Source: CAD feature listing. Evaluate the final solid. Frame: model axes, mm. A direction names the side the tool comes from. Round coordinates to 2 decimals unless told otherwise and drop trailing zeros. Write each loop counter-clockwise with the first axis right and the second up, starting at its lowest first coordinate (ties: lowest second). Pieces come first, ordered by that corner, then holes.
from build123d import *

# Parameters (mm, degrees)
SKETCH1_W           = 30
SKETCH1_H           = 10
BOSS_EXTRUDE1_DEPTH = 6.5
SKETCH3_W           = 13
SKETCH3_H           = 22
CUT_EXTRUDE3_DEPTH  = 20.163767897
SKETCH10_W          = 13
SKETCH10_H          = 10
BOSS_EXTRUDE3_DEPTH = 3
SKETCH12_W          = 22
SKETCH12_H          = 3.25
CUT_EXTRUDE5_DEPTH  = 0.5
SKETCH15_W          = 22
SKETCH15_H          = 3.375
BOSS_EXTRUDE6_DEPTH = 2


with BuildPart() as part:
    # Sketch1 → Boss-Extrude1 (new, symmetric)
    with BuildSketch(Plane.XY):
        Rectangle(SKETCH1_W, SKETCH1_H)
    extrude(amount=BOSS_EXTRUDE1_DEPTH, both=True)

    # Sketch3 → Cut-Extrude3 (cut, through all)
    with BuildSketch(Plane.XZ.offset(5)):
        with Locations((10.5, 0)):
            Rectangle(SKETCH3_W, SKETCH3_H)
    extrude(amount=-CUT_EXTRUDE3_DEPTH, mode=Mode.SUBTRACT)

    # Sketch10 → Boss-Extrude3 (add)
    with BuildSketch(Plane(origin=(4, 0, 0), x_dir=(0, 0, -1), z_dir=(1, 0, 0))):
        Rectangle(SKETCH10_W, SKETCH10_H)
    extrude(amount=BOSS_EXTRUDE3_DEPTH)

    # Sketch12 → Cut-Extrude5 (cut)
    with BuildSketch(Plane(origin=(0, 0, -6.5), x_dir=(-1, 0, 0), z_dir=(0, 0, -1))):
        with Locations((4, 0)):
            Rectangle(SKETCH12_W, SKETCH12_H)
    extrude(amount=-CUT_EXTRUDE5_DEPTH, mode=Mode.SUBTRACT)

    # Sketch15 → Boss-Extrude6 (add)
    with BuildSketch(Plane(origin=(0, 0, -6.5), x_dir=(-1, 0, 0), z_dir=(0, 0, -1))):
        with Locations((4, 3.3125)):
            Rectangle(SKETCH15_W, SKETCH15_H)
    boss_extrude6 = extrude(amount=BOSS_EXTRUDE6_DEPTH)

    # Mirror5: Boss-Extrude6 across plane
    add(boss_extrude6.mirror(Plane.ZX))


solid = part.part
1) Section query C-C on y = 0.25. Return the cut outline in (x, z).
Taken from the geometry:
outline: (-15, -6) - (7, -6) - (7, 6.5) - (-15, 6.5) - close
2) Section query A-A on z = -7. Return the cut outline in (x, y) (3 decimals), then the cut area to 4 significant figures.
Taken from the geometry:
outline: (-15, -5) - (7, -5) - (7, -1.625) - (-15, -1.625) - close; (-15, 1.625) - (7, 1.625) - (7, 5) - (-15, 5) - close
area: 148.5 mm2
3) Material intervals for line 1 (Y direction, x = 3.75, z = -6.5) (3 decimals); line 2 (Z direction, x = 5, y = 1.25), sorted ascending.
Taken from the geometry:
line 1: y = -5 to -1.625, 1.625 to 5
line 2: z = -6 to 6.5
4) Section query B-B on x = -1.5. Return the cut outline in (y, z) (3 decimals).
Taken from the geometry:
outline: (-5, -8.5) - (-1.625, -8.5) - (-1.625, -6) - (1.625, -6) - (1.625, -8.5) - (5, -8.5) - (5, 6.5) - (-5, 6.5) - close
5) Pull-direction query (Y, two-part tool) for faces 1 (the face through (-4, 5, -1)), 2 (the face through (-4, -3, -8.5)), 3 (the face through (-4, 0, -6)), 4 (the face through (-4, -1.625, -7)); classes: released by +Y, released by -Y, zero draft, split by the parting line, or undercut.
Taken from the geometry:
face 1: released by +Y
face 2: zero draft
face 3: undercut
face 4: undercut
6) Reachability of faces 5 (the face through (-4, 3, -8.5)), 6 (the face through (-4, 1.625, -7)) from +Z, -Z, +X, -X, +Y, -Y: full face, straight path, thin tool, end or side. Return the list, or none.
Taken from the geometry:
face 5: -Z, +X, -X, +Y, -Y
face 6: -Z, +X, -X
